Input: part model. Units: mm. Frame: model coordinates. A direction names the side the tool comes from. Coordinates: 2 decimals unless noted, no trailing zeros. Write each loop counter-clockwise with the first axis right and the second up, starting at its lowest first coordinate (ties: lowest second). Pieces come first, ordered by that corner, then holes. Notation, with made-up numbers: (9.25, -18.75) - (64.25, -18.75) arc R23 cw to (64.25, 12.25) - close; hole circle Ø4 at (30.5, 81.5). An arc over 180 degrees is marked (long way). Use a Markdown table: item, result. Add a question column.
Q1. Section query C-C (x = -22.5). Return the cut outline in (y, z), then the cut area to 3 significant figures.
Q2. Section query B-B (y = 12). Return the cut outline in (x, z), then the cut area to 3 significant figures.
Q3. Section query A-A (z = 12.5). Return the cut outline in (x, y).
Q4. Material intervals for probe 1 along X at (y, z) = (23.25, 12.5); probe 2 along Z at (x, y) = (-12.5, 23); probe 3 along Y at (x, z) = (-11, 4.25), sorted ascending. Write a range as from..to.
Q5. Mould query, pull axis Z, two halves, no side actions, for faces 3 (the face through (-13.974, 21.549, 11.148)), 4 (the face through (-15, 25, 12)), 5 (the face through (-20, 20, 25)). Classes: released by +Z, released by -Z, zero draft, split by the parting line, or undercut.
Q6. Set-up query: faces 1 (the face through (-25, 15, 12)), 2 (the face through (-18, 9, 13)). Return all of +Z, -Z, +X, -X, +Y, -Y with unobstructed straight access to the full face (end or side cutting, diameter ignored); none if empty.
Q7. Section query D-D (x = -14). Return the cut outline in (y, z), then the cut area to 3 significant figures.
Q8. Pin query (flat end, axial travel): P1, Ø5, axis at x = -18, z = 6, coming from the -Y side; P2, Ø8, axis at x = -3, y = 15.5, coming from the -Z side; P3, Ø12, axis at x = -15, y = 6, coming from the -Z side; P4, Ø3.5, axis at y = 12.5, z = 12.5, coming from the +X side. Return the tip coordinate at first contact, or that it passes through.
Autodesk Inventor part; units mm, degrees
ref_plane "YZ Plane" through (0, 0, 0) normal (1, 0, 0) x (0, 1, 0)
ref_plane "XZ Plane" through (0, 0, 0) normal (0, 1, 0) x (-1, 0, 0)
ref_plane "XY Plane" through (0, 0, 0) normal (0, 0, 1) x (1, 0, 0)
sketch "Sketch1" plane through (0, 0, 0) normal (0, 0, 1) x (1, 0, 0)
  line L0 (0, 0) -> (-25, 0)
  line L1 (-25, 0) -> (-25, 25)
  line L2 (-25, 25) -> (0, 25)
  line L3 (0, 25) -> (0, 0)
  dimension "d0" = 25
  dimension "d1" = 25
extrude "Extrusion1" add sketch "Sketch1" along normal blind 25
sketch "Sketch2" plane through (-25, 25, 0) normal (0, 1, 0) x (1, 0, 0)
  circle A0 centre (12.5, -12.5) radius 2
  line L0 (25, 0) -> (25, -25)
  line L1 (25, 0) -> (0, 0)
  arc A1 (12.5, -25) -> (12.5, 0) centre (12.5, -12.5) ccw
  line L2 (25, -25) -> (0, -25)
  point P0 (25, -12.5)
  dimension "d4" = 4
  dimension "d5" = 12.5
  dimension "d6" = 12.5
extrude "Extrusion2" cut sketch "Sketch2" against normal blind 25
sketch "Sketch3" plane through (0, 0, 25) normal (0, 0, 1) x (1, 0, 0)
  line L0 (0, 0) -> (-18, 0)
  line L1 (-18, 0) -> (-18, 18)
  line L2 (-18, 18) -> (0, 18)
  line L3 (0, 18) -> (0, 0)
  dimension "d9" = 18
  dimension "d10" = 18
extrude "Extrusion3" cut sketch "Sketch3" against normal blind 25
sketch "Sketch4" plane through (-18, 0, 25) normal (1, 0, 0) x (0, 0, -1)
  circle A0 centre (12.5, 12.5) radius 2
  line L0 (25, 0) -> (0, 0)
  line L1 (25, 18) -> (25, 0)
  arc A1 (0, 12.5) -> (25, 12.5) centre (12.5, 12.5) ccw
  line L2 (0, 0) -> (0, 18)
  point P0 (12.5, 0)
  dimension "d13" = 4
  dimension "d14" = 12.5
  dimension "d15" = 12.5
extrude "Extrusion4" cut sketch "Sketch4" against normal blind 25
properties part number "Frame Connector"
Values follow:
| question | item | result |
|---|---|---|
| 1 | outline | (12.5, 0) - (25, 0) - (25, 25) - (12.5, 25) arc R12.5 ccw to start; hole circle Ø4 at (12.5, 12.5) |
| 1 | area | 545 mm2 |
| 2 | outline | (-25, 0.01) - (-18, 0.01) - (-18, 10.56) - (-25, 10.56) - close; (-25, 14.44) - (-18, 14.44) - (-18, 24.99) - (-25, 24.99) - close |
| 2 | area | 148 mm2 |
| 3 | outline | (-25, 0) - (-18, 0) - (-18, 10.5) - (-25, 10.5) - close; (-25, 14.5) - (-18, 14.5) - (-18, 18) - (-14.5, 18) - (-14.5, 25) - (-25, 25) - close; (-10.5, 18) - (0, 18) - (0, 25) - (-10.5, 25) - close |
| 4 | probe 1 | -25..-14.5, -10.5..0 |
| 4 | probe 2 | 0..10.5, 14.5..25 |
| 4 | probe 3 | 18..25 |
| 5 | face 3 | undercut |
| 5 | face 4 | zero draft |
| 5 | face 5 | released by +Z |
| 6 | face 1 | +Z, -Z, -X, +Y, -Y |
| 6 | face 2 | +Z, -Z, +X, -Y |
| 7 | outline | (18, 0) - (25, 0) - (25, 11.18) - (18, 11.18) - close; (18, 13.82) - (25, 13.82) - (25, 25) - (18, 25) - close |
| 7 | area | 156 mm2 |
| 8 | P1 | y = 0.66 |
| 8 | P2 | z = 1.75 |
| 8 | P3 | z = 0.07 |
| 8 | P4 | through |
